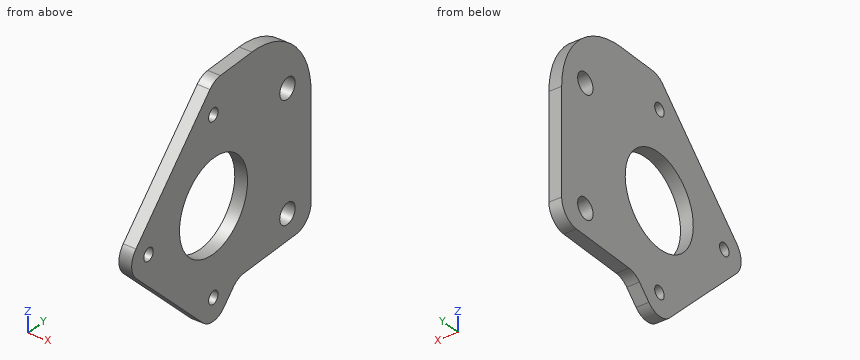
from build123d import *

# Parameters (mm, degrees)
BASE_FLANGE1_DEPTH             = 3.175
F_23_0_23_DIAMETER_HOLE1_D     = 23
F_23_0_23_DIAMETER_HOLE1_DEPTH = 5.245059642
F_5_2_5_2_DIAMETER_HOLE1_D     = 5.2
F_5_2_5_2_DIAMETER_HOLE1_DEPTH = 5.245059642
F_3_2_3_2_DIAMETER_HOLE1_D     = 3.2
F_3_2_3_2_DIAMETER_HOLE1_DEPTH = 5.245059642


# Sheet-metal steps are written as plain solids
with BuildPart() as part:
    # Sketch11 → Base-Flange1 (new body)
    with BuildSketch(Plane(origin=(158.683156088, 5.425207604, 0), x_dir=(0.03416896788300158, -0.9994160703299755, 0), z_dir=(-0.9994160703299755, -0.03416896788300158, -1.3885688057658037e-15))):
        with BuildLine():
            Line((-62.15623968, 394.926215189), (-62.15623968, 368.398551724))
            ThreePointArc((-62.15623968, 368.398551724), (-60.691773586, 364.863017818), (-57.15623968, 363.398551724))
            Line((-57.15623968, 363.398551724), (-39.397236161, 363.398551724))
            ThreePointArc((-39.397236161, 363.398551724), (-37.483818999, 363.017949386), (-35.861702255, 361.93408563))
            Line((-35.861702255, 361.93408563), (-32.700762633, 358.773146007))
            ThreePointArc((-32.700762633, 358.773146007), (-29.165228727, 357.308679913), (-25.629694821, 358.773146007))
            Line((-25.629694821, 358.773146007), (-3.002277823, 381.400563005))
            ThreePointArc((-3.002277823, 381.400563005), (-1.537811729, 384.936096911), (-3.002277823, 388.471630817))
            Line((-3.002277823, 388.471630817), (-27.992396101, 413.461749095))
            ThreePointArc((-27.992396101, 413.461749095), (-29.614512845, 414.545612852), (-31.527930007, 414.926215189))
            Line((-31.527930007, 414.926215189), (-42.15623968, 414.926215189))
            ThreePointArc((-42.15623968, 414.926215189), (-56.298375303, 409.068350813), (-62.15623968, 394.926215189))
        make_face()
    extrude(amount=-BASE_FLANGE1_DEPTH)

    # Ø23.0 (23) Diameter Hole1
    with Locations(Plane(origin=(158.683156088, 5.425207604, 0), x_dir=(0, 0, 1), z_dir=(-0.9994160703299755, -0.03416896788300158, -1.3885688057658039e-15))):
        with Locations((384.926215189, 29.191594771)):
            Hole(F_23_0_23_DIAMETER_HOLE1_D / 2, depth=F_23_0_23_DIAMETER_HOLE1_DEPTH)

    # Ø5.2 (5.2) Diameter Hole1
    with Locations(Plane(origin=(158.683156088, 5.425207604, 0), x_dir=(0, 0, 1), z_dir=(-0.9994160703299755, -0.03416896788300158, -1.3885688057658039e-15))):
        with Locations((369.898551724, 54.15623968), (399.898551724, 54.15623968)):
            Hole(F_5_2_5_2_DIAMETER_HOLE1_D / 2, depth=F_5_2_5_2_DIAMETER_HOLE1_DEPTH)

    # Ø3.2 (3.2) Diameter Hole1
    with Locations(Plane(origin=(158.683156088, 5.425207604, 0), x_dir=(0, 0, 1), z_dir=(-0.9994160703299755, -0.03416896788300158, -1.3885688057658039e-15))):
        with Locations((406.806051724, 29.127683539), (362.991051724, 29.127683539), (384.898551724, 7.220183539)):
            Hole(F_3_2_3_2_DIAMETER_HOLE1_D / 2, depth=F_3_2_3_2_DIAMETER_HOLE1_DEPTH)


solid = part.part
Check sheet for the modelled part. Datum: model origin and axes. Units: mm. Coordinates: 2 decimals unless noted, no trailing zeros. Loops run counter-clockwise (first coordinate to the right, second up) from the corner with the lowest first, then second, coordinate; pieces in that order, holes last. Notation, with made-up numbers: (65.25, 43.25) -> (90.25, 43.25) arc R7 cw to (90.25, 55.25) -> close; hole circle Ø5 at (13, 87.5). An arc over 180 degrees is marked (long way). Answer in a Markdown table with one row per item.
1. Go/stop test with flat-tipped pins: pin 1 (1 mm diameter, centred on y = 48, z = 406.5, fed in from +X); pin 2 (1 mm diameter, centred on y = 52.5, z = 365.5, fed in from +X); pin 3 (1.9 mm diameter, centred on x = 159, y = 56, fed in from -Z). Record where each tip stops, or that it passes through.
Check values:
| item | result |
|---|---|
| pin 1 | stops at x = 160.42 |
| pin 2 | stops at x = 160.27 |
| pin 3 | stops at z = 363.4 |
2. Sectioned sample at B-B, the plane z = 366. Record the boundary of the cut face in (x, y).
Check values:
| item | result |
|---|---|
| outline | (156.58, 66.93) -> (158.05, 23.82) -> (161.23, 23.93) -> (159.75, 67.04) -> close |
3. Material ranges on line 1 along Z through (x, y) = (157.1, 60); line 2 along Z through (x, y) = (159.35, 31); line 3 along Z through (x, y) = (161.1, 20.5), recorded low to high. Write a range as [from, to].
Check values:
| item | result |
|---|---|
| line 1 | z = [363.4, 367.34], [372.46, 397.34], [402.46, 410.59] |
| line 2 | z = [358.87, 374.02], [395.83, 411.01] |
| line 3 | z = [369.42, 400.45] |
4. Sectioned sample at A-A, the plane y = 61. Give the number of separate pieces and of enclosed holes in the cut face, then the cut area to 3 significant figures.
Check values:
| item | result |
|---|---|
| separate pieces | 3 |
| enclosed holes | 0 |
| area | 119 mm2 |
